Source: CAD feature listing. Evaluate the final solid. Frame: model axes, mm. Round coordinates to 2 decimals unless told otherwise and drop trailing zeros. Write each loop counter-clockwise with the first axis right and the second up, starting at its lowest first coordinate (ties: lowest second). Pieces come first, ordered by that corner, then holes. Notation, with made-up numbers: M -1.75,-14 L 4.25,-14 A13 ccw 4.25,-1 Z; hole C -2,35 d8. An arc over 180 degrees is marked long. Use a Markdown table: item, result.
```python
from build123d import *

# Parameters (mm, degrees)
F0_R     = 9.65
F1_DEPTH = 5
F3_DEPTH = 5.001


with BuildPart() as f1:
    # F0 (on Top) → F1 (new body)
    with BuildSketch(Plane.XY):
        Circle(F0_R)
    extrude(amount=F1_DEPTH)

    # F2 (on face) → F3 (cut, through all)
    with BuildSketch(Plane.XY.offset(5)):
        with BuildLine():
            ThreePointArc((2.3027162866, 4.4381863079), (2.0398793124, 1.311303699), (4.9936375982, 0.252157763))
            ThreePointArc((4.9936375982, 0.252157763), (4.2059367266, 2.7037189669), (2.3027162866, 4.4381863079))
        make_face()
        with BuildLine():
            ThreePointArc((2.3027162866, 4.4381863079), (4.2059367266, 2.7037189669), (4.9936375982, 0.252157763))
            ThreePointArc((4.9936375982, 0.252157763), (6.286676348, 1.1867655636), (6.7809367266, 2.7037189669))
            ThreePointArc((6.7809367266, 2.7037189669), (5.1359454274, 5.1049080091), (2.3027162866, 4.4381863079))
        make_face()
        with BuildLine():
            ThreePointArc((2.8135209468, -4.9943075354), (2.783016007, -4.5991241749), (2.692223946, -4.2133039558))
            ThreePointArc((2.692223946, -4.2133039558), (0.2385209468, -4.9943075354), (-2.2784437706, -4.4506958988))
            ThreePointArc((-2.2784437706, -4.4506958988), (-0.0348294261, -7.5547576079), (2.8135209468, -4.9943075354))
        make_face()
        with BuildLine():
            ThreePointArc((-2.2784437706, -4.4506958988), (0.2385209468, -4.9943075354), (2.692223946, -4.2133039558))
            ThreePointArc((2.692223946, -4.2133039558), (0.1156826592, -2.4222391547), (-2.2784437706, -4.4506958988))
        make_face()
        with BuildLine():
            ThreePointArc((-1.8694576733, 2.2905885685), (-2.090367679, 3.3340852377), (-2.7151938276, 4.1985381359))
            ThreePointArc((-2.7151938276, 4.1985381359), (-4.4444576733, 2.2905885685), (-4.9949402326, -0.224882352))
            ThreePointArc((-4.9949402326, -0.224882352), (-2.8299713139, 0.2845828867), (-1.8694576733, 2.2905885685))
        make_face()
        with BuildLine():
            ThreePointArc((-4.9949402326, -0.224882352), (-4.4444576733, 2.2905885685), (-2.7151938276, 4.1985381359))
            ThreePointArc((-2.7151938276, 4.1985381359), (-6.7333533751, 3.4702416812), (-4.9949402326, -0.224882352))
        make_face()
    extrude(amount=-F3_DEPTH, mode=Mode.SUBTRACT)


solid = f1.part
```
Q1. Line query: L1, parallel to X at y = 2.75, z = 4.6; L2, parallel to Y at x = 2.5, z = 3.75; L3, parallel to Y at x = -1.25, z = 1.1. Output: solid intervals per line, ascending.
Results are:
| item | result |
|---|---|
| L1 | -9.25 to -6.98, -1.91 to 1.63, 6.78 to 9.25 |
| L2 | -9.32 to -6.23, -3.76 to 0.77, 4.63 to 9.32 |
| L3 | -9.57 to -7.1, -2.89 to 9.57 |
Q2. Section D-D on x = -8. Return loops of the section in (y, z), plus the area to 3 significant figures.
Results are:
| item | result |
|---|---|
| outline | M -5.4,0 L 5.4,0 L 5.4,5 L -5.4,5 Z |
| area | 54.0 mm^2 |
Q3. Section B-B on y = -6. Return loops of the section in (x, z), plus the area to 3 significant figures.
Results are:
| item | result |
|---|---|
| outline | M -7.56,0 L -2.13,0 L -2.13,5 L -7.56,5 Z; M 2.61,0 L 7.56,0 L 7.56,5 L 2.61,5 Z |
| area | 51.9 mm^2 |
Q4. Section C-C on y = 5.75. Return loops of the section in (x, z).
Results are:
| item | result |
|---|---|
| outline | M -7.75,0 L 7.75,0 L 7.75,5 L -7.75,5 Z |
Q5. Section A-A on x = 3.75. Return loops of the section in (y, z), plus the area to 3 significant figures.
Results are:
| item | result |
|---|---|
| outline | M -8.89,0 L 0.17,0 L 0.17,5 L -8.89,5 Z; M 5.24,0 L 8.89,0 L 8.89,5 L 5.24,5 Z |
| area | 63.6 mm^2 |
Q6. First-contact query: pin 1 Ø2 at (y, z) = (4, 3) entering from +X; pin 2 Ø4.5 at (x, y) = (-4.44, 2.29) entering from +Z; pin 3 Ø8 at (x, y) = (0.24, -4.99) entering from -Z; pin 4 Ø1.5 at (y, z) = (3, 0.5) entering from -X. Flat tips, straight axial feed; report the tip coordinate or a pass-through.
Results are:
| item | result |
|---|---|
| pin 1 | x = 9.17 |
| pin 2 | through |
| pin 3 | z = 0 |
| pin 4 | x = -9.38 |
